Can you work these out from the model? Positions are in its coordinate system, mm. A direction names the side the tool comes from. Give positions to 0.01 mm unless a question says otherwise; leave off trailing zeros. Write each loop counter-clockwise with the first axis right and the second up, starting at its lowest first coordinate (ties: lowest second). Pieces come first, ordered by that corner, then holes.
from build123d import *

# Parameters (mm, degrees)
EXTRUDE_1_DEPTH             = 30
SKETCH_5_R                  = 20
CUT_EXTRUDE_1_DEPTH         = 15
SKETCH_6_R                  = 5
CUT_EXTRUDE_2_DEPTH         = 109.397416943
FILLET_1_R                  = 6
SKETCH_7_R                  = 15
CUT_EXTRUDE_3_DEPTH         = 15
HOLE_WIZARD_M62_D           = 6.6
HOLE_WIZARD_M62_CSINK_D     = 8
HOLE_WIZARD_M62_CSINK_ANGLE = 90
PATTERN_LINEAR_1_COUNT      = 2
PATTERN_LINEAR_1_PITCH      = 18
PATTERN_LINEAR_1_COUNT_DIR2 = 2
PATTERN_LINEAR_1_PITCH_DIR2 = 84
FILLET_2_R                  = 3


with BuildPart() as part:
    # Эскиз4 → Бобышка-Вытянуть1 (new body)
    with BuildSketch(Plane.XY):
        with BuildLine():
            Line((0, 0), (50, 0))
            Line((50, 0), (50, 10))
            Line((50, 10), (10, 10))
            ThreePointArc((10, 10), (20.916500663, 19.219814537), (25, 32.912878475))
            Line((25, 32.912878475), (25, 70))
            ThreePointArc((25, 70), (17.67766953, 87.67766953), (0, 95))
            Line((0, 95), (0, 0))
        make_face()
    extrude_1 = extrude(amount=-EXTRUDE_1_DEPTH)

    # Зеркальное отражение1: Бобышка-Вытянуть1 across plane
    add(extrude_1.mirror(Plane(origin=(0, 0, -30), x_dir=(0, 0, 1), z_dir=(-1, 0, 0))))

    # Эскиз5 → Вырез-Вытянуть1 (cut)
    with BuildSketch(Plane.XY):
        with Locations((0, 70)):
            Circle(SKETCH_5_R)
    extrude(amount=-CUT_EXTRUDE_1_DEPTH, mode=Mode.SUBTRACT)

    # Эскиз6 → Вырез-Вытянуть2 (cut, through all)
    with BuildSketch(Plane.XY.offset(-15)):
        with Locations((0, 70)):
            Circle(SKETCH_6_R)
    extrude(amount=-CUT_EXTRUDE_2_DEPTH, mode=Mode.SUBTRACT)

    # Скругление1
    fillet_1_edges = [part.edges().sort_by_distance(p)[0] for p in [
        (10, 10, -15),
        (-10, 10, -15),
    ]]
    fillet(fillet_1_edges, radius=FILLET_1_R)

    # Эскиз7 → Вырез-Вытянуть3 (cut)
    with BuildSketch(Plane.XY):
        with Locations((0, 42.5)):
            Circle(SKETCH_7_R)
    extrude(amount=-CUT_EXTRUDE_3_DEPTH, mode=Mode.SUBTRACT)

    # Зенковка для винта с полупотайной головкой M62 (through all)
    with Locations(Plane(origin=(42, 10, -24), x_dir=(1, 0, 0), z_dir=(0, 1, 0))):
        with Locations((0, 0)):
            hole_wizard_m62 = CounterSinkHole(HOLE_WIZARD_M62_D / 2, HOLE_WIZARD_M62_CSINK_D / 2, counter_sink_angle=HOLE_WIZARD_M62_CSINK_ANGLE)

    # Линейный массив1: Hole Wizard M62 2 × 2
    with Locations(*[(-j * PATTERN_LINEAR_1_PITCH_DIR2, 0, i * PATTERN_LINEAR_1_PITCH) for i in range(PATTERN_LINEAR_1_COUNT) for j in range(PATTERN_LINEAR_1_COUNT_DIR2) if (i, j) != (0, 0)]):
        add(hole_wizard_m62, mode=Mode.SUBTRACT)

    # Скругление2
    fillet_2_edges = [part.edges().sort_by_distance(p)[0] for p in [
        (50, 5, -30),
        (-50, 5, 0),
        (-50, 5, -30),
        (50, 5, 0),
    ]]
    fillet(fillet_2_edges, radius=FILLET_2_R)


solid = part.part
(1) Imagine slicing it at B-B, the plane y = 42.5. Write out the boundary of the cut face in (x, z).
Returned:
outline: (-25, -30) - (25, -30) - (25, 0) - (15, 0) - (15, -15) - (-15, -15) - (-15, 0) - (-25, 0) - close
(2) Will these pins go through, and if not, where does the flat tip stop? P1, Ø9, axis at y = 59, z = -15.5, coming from the +X side; P2, Ø3, axis at x = 12, z = -16.5, coming from the +Y side; P3, Ø12, axis at x = -41.5, z = -11.5, coming from the +Y side.
Returned:
P1: stops at x = 25
P2: stops at y = 92.69
P3: stops at y = 10
(3) Imagine slicing it at A-A, the plane x = 42. Write out the boundary of the cut face in (y, z).
Returned:
outline: (0, -30) - (10, -30) - (10, -28) - (9.3, -27.3) - (0, -27.3) - close; (0, -20.7) - (9.3, -20.7) - (10, -20) - (10, -10) - (9.3, -9.3) - (0, -9.3) - close; (0, -2.7) - (9.3, -2.7) - (10, -2) - (10, 0) - (0, 0) - close
(4) Imagine slicing it at D-D, the plane z = -25.5. Give the number of separate pieces and of enclosed holes in the cut face, plus the area to 3 significant figures.
Returned:
separate pieces: 3
enclosed holes: 1
area: 4,670 mm2
(5) For faces 1 (the face through (-49.1, 5.07, -29.14)), 2 (the face through (0.722, 89.987, -7.395)), 3 (the face through (23.938, 25.702, -14.79)), which set-ups out of +Z, -Z, +X, -X, +Y, -Y let a thin tool reach every point of the face, with its end or its side?
Returned:
face 1: -Z, -X, +Y, -Y
face 2: +Z
face 3: +Z, -Z, +X
(6) Imagine slicing it at C-C, the plane z = -18.75. Write out the boundary of the cut face in (x, y), plus the area to 3 significant figures.
Returned:
outline: (-50, 0) - (50, 0) - (50, 10) - (25.98, 10) arc R6 cw to (20.95, 19.27) arc R25 ccw to (25, 32.91) - (25, 70) arc R25 ccw to (-25, 70) - (-25, 32.91) arc R25 ccw to (-20.95, 19.27) arc R6 cw to (-25.98, 10) - (-50, 10) - close; hole circle Ø10 at (0, 70)
area: 4,790 mm2
(7) If I drill on L1, parallel to Z at x = -42, y = 2.5; L2, parallel to X at y = 4.5, z = -24; L3, parallel to Y at x = 0, z = -22.5, over which ranges is the centre line in solid material (lowest first)?
Returned:
L1: z = -30 to -27.3, -20.7 to -9.3, -2.7 to 0
L2: x = -50 to -45.3, -38.7 to 38.7, 45.3 to 50
L3: y = 0 to 65, 75 to 95
(8) If we mould it in two halves opening along X, with no side actions, what happens to faces 4 (the face through (-20.75, 13.06, -15.21)), 5 (the face through (-38.7, 4.6, -6.1)), 6 (the face through (1, 48, -30)), 7 (the face through (49.1, 5.07, -29.14))? For each: +X half, -X half, draft (parallel to the pull), parting line (faces both ways), or undercut.
Returned:
face 4: -X half
face 5: undercut
face 6: draft
face 7: +X half
